Design review of the part built by this model. Coordinates are the model's own, in mm. A direction names the side the tool comes from. Give positions to 0.01 mm unless a question says otherwise; leave off trailing zeros. Loops run counter-clockwise (first coordinate to the right, second up) from the corner with the lowest first, then second, coordinate; pieces in that order, holes last. Notation, with made-up numbers: (44.5, -30.75) - (50.5, -30.75) arc R22 cw to (50.5, -1.75) - close; hole circle Ø4 at (42.5, 85). An arc over 180 degrees is marked (long way). Put each result on its own line as item: value. Start each with the question number.
```python
from build123d import *

# Parameters (mm, degrees)
BASPROSKE_W              = 8
BASPROSKE_H              = 30
TOOTHCUT_DEPTH           = 44.17406629
TEETHCUTS_COUNT          = 28
TEETHCUTS_ANGLE          = 347.142857143
BORSKE_R                 = 0.1
BORE_DEPTH               = 50.0000508
TAGLIO_ESTRUSIONE1_DEPTH = 30
SCHIZZO2_R               = 1.6
TAGLIO_ESTRUSIONE2_DEPTH = 10
SCHIZZO3_R               = 11
TAGLIO_ESTRUSIONE3_DEPTH = 2


with BuildPart() as part:
    # BasProSke → Base-Revolve (revolve)
    with BuildSketch(Plane(origin=(0, 0, 0), x_dir=(1, 0, 0), z_dir=(0, 1, 0)), mode=Mode.PRIVATE) as base_revolve_sk:
        with Locations((4, 15)):
            Rectangle(BASPROSKE_W, BASPROSKE_H)
    revolve(base_revolve_sk.sketch.rotate(Axis((-10, 0, 0), (1, 0, 0)), 180), axis=Axis((-10, 0, 0), (1, 0, 0)))

    # TooCutSke → ToothCut (cut, through all)
    with BuildSketch(Plane(origin=(0, 0, 0), x_dir=(0, 0, -1), z_dir=(1, 0, 0))):
        with BuildLine():
            ThreePointArc((0.928503763, 25.482089431), (0, 25.499), (-0.928503763, 25.482089431))
            ThreePointArc((-0.928503763, 25.482089431), (-1.618524429, 27.789411612), (-2.78585155, 29.895880591))
            ThreePointArc((-2.78585155, 29.895880591), (0, 30.0254), (2.78585155, 29.895880591))
            ThreePointArc((2.78585155, 29.895880591), (1.618524429, 27.789411612), (0.928503763, 25.482089431))
        make_face()
    toothcut = extrude(amount=TOOTHCUT_DEPTH, mode=Mode.SUBTRACT)

    # TeethCuts: ToothCut ×28 about axis
    teethcuts_axis = Axis((-10, 0, 0), (1, 0, 0))
    for i in range(1, TEETHCUTS_COUNT):
        add(toothcut.rotate(teethcuts_axis, i * TEETHCUTS_ANGLE / (TEETHCUTS_COUNT - 1)), mode=Mode.SUBTRACT)

    # BorSke → Bore (cut, symmetric)
    with BuildSketch(Plane(origin=(0, 0, 0), x_dir=(0, 0, -1), z_dir=(1, 0, 0))):
        with Locations(Location((0, 0, 0), (0, 0, 180))):
            Circle(BORSKE_R)
    extrude(amount=BORE_DEPTH, both=True, mode=Mode.SUBTRACT)

    # Schizzo1 → Taglio-Estrusione1 (cut)
    with BuildSketch(Plane(origin=(8, 0, 0), x_dir=(0, 0, -1), z_dir=(1, 0, 0))):
        with BuildLine():
            Line((-1.5, 2), (1.5, 2))
            ThreePointArc((1.5, 2), (0, -2.5), (-1.5, 2))
        make_face()
    extrude(amount=-TAGLIO_ESTRUSIONE1_DEPTH, mode=Mode.SUBTRACT)

    # Schizzo2 → Taglio-Estrusione2 (cut)
    with BuildSketch(Plane.ZY):
        with Locations((0, 8)):
            Circle(SCHIZZO2_R)
        with Locations((8, 0)):
            Circle(SCHIZZO2_R)
        with Locations((0, -8)):
            Circle(SCHIZZO2_R)
        with Locations((-8, 0)):
            Circle(SCHIZZO2_R)
    extrude(amount=-TAGLIO_ESTRUSIONE2_DEPTH, mode=Mode.SUBTRACT)

    # Schizzo3 → Taglio-Estrusione3 (cut)
    with BuildSketch(Plane(origin=(8, 0, 0), x_dir=(0, 0, -1), z_dir=(1, 0, 0))):
        Circle(SCHIZZO3_R)
    extrude(amount=-TAGLIO_ESTRUSIONE3_DEPTH, mode=Mode.SUBTRACT)


solid = part.part
```
Item 1: Consider section B-B (y = 0). State the section outline as (x, z) points.
Item 2: Consider section C-C (y = -8). State the section outline as (x, z) points.
Item 3: Mouldability with a two-part tool opening along Z and no side actions: class faces 4 (the cylindrical face through (3.944, -7.773, -26.748)), 5 (the cylindrical face through (3.94, 25.76, 10.6)) as pulls with the +Z half, pulls with the -Z half, needs draft (parallel to the pull), parting line crosses it, or undercut.
Item 4: For P1, Ø4, axis at y = 9.5, z = -1, coming from the -X side; P2, Ø4, axis at y = -8, z = 0, coming from the +X side; P3, Ø2, axis at x = 2, y = 8, coming from the -Z side, all flat-tipped, find the tip position at first contact; note any pin that passes through.
Item 5: Consider section D-D (x = 1). Count the separate pieces of the cut face and the enclosed holes in it, plus the area to 3 significant figures.
Item 6: Machinability: for faces 1 (the cylindrical face through (3.94, 26.69, 7.73)), 2 (the cylindrical face through (3.944, -19.944, -15.888)), 3 (the cylindrical face through (3.944, -24.863, -5.661)), which of the approach directions +Z, -Z, +X, -X, +Y, -Y give a long, thin tool a straight path to every point of the face, cutting with its end or side? Answer none if there is none.
Item 7: Consider section A-A (z = 0). State the section outline as (x, y) points.
Item 8: For L1, parallel to Y at x = 3.65, z = 0; L2, parallel to Y at x = 1.75, z = -23.5; L3, parallel to Z at x = 1, y = -26, list the stretches that pass through material, from the lowest coordinate up. Write a range as from..to.
Geometry says:
1. outline: (0, -25.5) - (8, -25.5) - (8, -11) - (6, -11) - (6, -9.6) - (0, -9.6) - close; (0, -6.4) - (6, -6.4) - (6, -2.5) - (0, -2.5) - close; (0, 2.5) - (6, 2.5) - (6, 6.4) - (0, 6.4) - close; (0, 9.6) - (6, 9.6) - (6, 11) - (8, 11) - (8, 25.5) - (0, 25.5) - close
2. outline: (0, -27.05) - (8, -27.05) - (8, -7.55) - (6, -7.55) - (6, -1.6) - (0, -1.6) - close; (0, 1.6) - (6, 1.6) - (6, 7.55) - (8, 7.55) - (8, 27.05) - (0, 27.05) - close
3. face 4: pulls with the -Z half
3. face 5: undercut
4. P1: stops at x = 0
4. P2: stops at x = 6
4. P3: stops at z = -28.18
5. separate pieces: 1
5. enclosed holes: 5
5. area: 2,360 mm2
6. face 1: +X, -X, +Y
6. face 2: +X, -X
6. face 3: +X, -X, -Y
7. outline: (0, -25.5) - (8, -25.5) - (8, -11) - (6, -11) - (6, -9.6) - (0, -9.6) - close; (0, -6.4) - (6, -6.4) - (6, -2.5) - (0, -2.5) - close; (0, 2) - (6, 2) - (6, 6.4) - (0, 6.4) - close; (0, 9.6) - (6, 9.6) - (6, 11) - (8, 11) - (8, 25.5) - (0, 25.5) - close
8. L1: y = -25.5..-9.6, -6.4..-2.5, 2..6.4, 9.6..25.5
8. L2: y = -16.25..-12.67, -10.26..10.26, 12.67..16.25
8. L3: z = -10.61..-7.28, -4.76..-1.04, 1.04..4.76, 7.28..10.61
